```python
from build123d import *

# Parameters (mm, degrees)
CROQUIS2_R            = 4
CORTAR_EXTRUIR1_DEPTH = 51.449231907
REDONDEO1_R           = 4


with BuildPart() as part:
    # Croquis1 → Revolución1 (revolve)
    with BuildSketch(Plane.XY, mode=Mode.PRIVATE) as revoluci_n1_sk:
        Polygon((0, 0), (0, 19.5), (5, 19.5), (5, 31.75), (-15, 31.75), (-15, 19.5), (-18, 10), (-18, 0), align=None)
    revolve(revoluci_n1_sk.sketch.rotate(Axis((-18, 0, 0), (1, 0, 0)), 180), axis=Axis((-18, 0, 0), (1, 0, 0)))

    # Croquis2 → Cortar-Extruir1 (cut, through all)
    with BuildSketch(Plane.ZY.offset(18)):
        with Locations(Location((0, 0, 0), (0, 0, 270))):
            Circle(CROQUIS2_R)
    extrude(amount=-CORTAR_EXTRUIR1_DEPTH, mode=Mode.SUBTRACT)

    # Redondeo1
    redondeo1_edges = [part.edges().sort_by_distance(p)[0] for p in [
        (-15, 31.75, 0),
        (5, 31.75, 0),
    ]]
    fillet(redondeo1_edges, radius=REDONDEO1_R)


solid = part.part
```
Geometry: final body of the model. Coordinates: model frame, mm. A direction names the side the tool comes from. Give positions to 0.01 mm unless a question says otherwise; leave off trailing zeros. Loops run counter-clockwise (first coordinate to the right, second up) from the corner with the lowest first, then second, coordinate; pieces in that order, holes last. Notation, with made-up numbers: (2.25, 34) -> (10.25, 34) arc R15 ccw to (10.25, 58) -> close; hole circle Ø10 at (72, 20). An arc over 180 degrees is marked (long way). Use CSV: the item, a comma, the result in double quotes.
(1) Cut plane D-D (x = 2.75). Output: boundary loops of the cut face in (y, z), plus the area to 3 significant figures.
From the geometry:
outline,"circle Ø62.69 at (0, 0); hole circle Ø39 at (0, 0)"
area,"1,890 mm^2"
(2) Cut plane A-A (z = 0). Output: boundary loops of the cut face in (x, y).
From the geometry:
outline,"(-18, -10) -> (-15, -19.5) -> (-15, -27.75) arc R4 ccw to (-11, -31.75) -> (1, -31.75) arc R4 ccw to (5, -27.75) -> (5, -19.5) -> (0, -19.5) -> (0, -4) -> (-18, -4) -> close; (-18, 4) -> (0, 4) -> (0, 19.5) -> (5, 19.5) -> (5, 27.75) arc R4 ccw to (1, 31.75) -> (-11, 31.75) arc R4 ccw to (-15, 27.75) -> (-15, 19.5) -> (-18, 10) -> close"
(3) Cut plane C-C (x = -4.75). Output: boundary loops of the cut face in (y, z).
From the geometry:
outline,"circle Ø63.5 at (0, 0); hole circle Ø8 at (0, 0)"
(4) Pull-direction query (Z, two-part tool) for faces 3 (the face through (0, 0, -5)), 4 (the face through (-17.854, -9.978, -3.142)), 5 (the face through (-9.126, 0.867, -3.905)), 6 (the face through (-15, -6, -19)); classes: released by +Z, released by -Z, zero draft, split by the parting line, or undercut.
From the geometry:
face 3,"undercut"
face 4,"split by the parting line"
face 5,"undercut"
face 6,"zero draft"
(5) Ray query, line 1 along X through (y, z) = (-13, 14.5); line 2 along X through (y, z) = (23, -9); line 3 along Y through (x, z) = (-11.5, -3.5). Return the intervals inside material, ascending. Write a range as [from, to].
From the geometry:
line 1,"[-15.01, 0]"
line 2,"[-15, 5]"
line 3,"[-31.52, -1.94], [1.94, 31.52]"
(6) Access query for faces 1 (the face through (5, 6, -19)), 2 (the face through (2.535, 2.539, -19.334)). Directions: +Z, -Z, +X, -X, +Y, -Y. A direction counts if a zero-diameter tool reaches every point of the face in a straight line with its end or side. Return the directions, or none.
From the geometry:
face 1,"+Z, -Z, +X, +Y, -Y"
face 2,"+X"
(7) First-contact query: P1, Ø1, axis at x = 0, z = -8.5, coming from the -Y side; P2, Ø11.5, axis at y = -8.5, z = -8, coming from the +X side; P3, Ø2, axis at x = -14.5, y = 6.5, coming from the +Z side. Flat tips, straight axial feed; report the tip coordinate or a pass-through.
From the geometry:
P1,"y = -30.73"
P2,"x = 0"
P3,"z = 30.21"
